Verification items for the finished model (mm, model axes). A direction names the side the tool comes from. Coordinates: 2 decimals unless noted, no trailing zeros. Write each loop counter-clockwise with the first axis right and the second up, starting at its lowest first coordinate (ties: lowest second). Pieces come first, ordered by that corner, then holes. Notation, with made-up numbers: M 29,-15.75 L 38,-15.75 A21 ccw 38,1.25 Z; hole C 70,29.5 d9. An arc over 180 degrees is marked long. Answer in a Markdown table with one row per item.
from build123d import *

# Parameters (mm, degrees)
SKETCH1_W           = 139.7
SKETCH1_H           = 12.7
BOSS_EXTRUDE1_DEPTH = 101.6
SKETCH2_W           = 12.7
SKETCH2_H           = 6.35
BOSS_EXTRUDE2_DEPTH = 19.05
CUT_EXTRUDE1_REACH  = 190.906
SKETCH3_R           = 5.207
SKETCH4_R           = 22.225
CUT_EXTRUDE2_DEPTH  = 11.43
CUT_EXTRUDE3_REACH  = 190.825
SKETCH5_R           = 1.7018
SKETCH5_R_2         = 2.2479
CUT_EXTRUDE4_REACH  = 187.568
SKETCH6_R           = 3.175
FILLET1_R           = 2.54


with BuildPart() as part:
    # Sketch1 → Boss-Extrude1 (new body)
    with BuildSketch(Plane(origin=(0, 0, 0), x_dir=(1, 0, 0), z_dir=(0, 1, 0))):
        with Locations((69.85, 6.35)):
            Rectangle(SKETCH1_W, SKETCH1_H)
    extrude(amount=BOSS_EXTRUDE1_DEPTH)

    # Sketch2 → Boss-Extrude2 (add)
    with BuildSketch(Plane.ZY):
        with Locations((-6.35, 3.175)):
            Rectangle(SKETCH2_W, SKETCH2_H)
    boss_extrude2 = extrude(amount=BOSS_EXTRUDE2_DEPTH)

    # Mirror1: Boss-Extrude2 across plane
    add(boss_extrude2.mirror(Plane.ZY.offset(-69.85)))

    # Sketch3 → Cut-Extrude1 (cut, up to next)
    with BuildSketch(Plane.XY, mode=Mode.PRIVATE) as cut_extrude1_sk1:
        with Locations((69.85, 76.2)):
            Circle(SKETCH3_R)
    cut_extrude1_tool1 = extrude(cut_extrude1_sk1.sketch, amount=-CUT_EXTRUDE1_REACH, mode=Mode.PRIVATE) & part.part
    add(cut_extrude1_tool1.solids().sort_by_distance((69.85, 76.2, 0))[0], mode=Mode.SUBTRACT)

    # Sketch4 → Cut-Extrude2 (cut)
    with BuildSketch(Plane.XY):
        with Locations((69.85, 76.2)):
            Circle(SKETCH4_R)
    extrude(amount=-CUT_EXTRUDE2_DEPTH, mode=Mode.SUBTRACT)

    # Sketch5 → Cut-Extrude3 (cut, up to next)
    with BuildSketch(Plane.XY.offset(-11.43), mode=Mode.PRIVATE) as cut_extrude3_sk1:
        with Locations((58.851477372, 82.55)):
            Circle(SKETCH5_R)
    cut_extrude3_tool1 = extrude(cut_extrude3_sk1.sketch, amount=-CUT_EXTRUDE3_REACH, mode=Mode.PRIVATE) & part.part
    # Sketch5 → Cut-Extrude3 (cut, up to next)
    with BuildSketch(Plane.XY.offset(-11.43), mode=Mode.PRIVATE) as cut_extrude3_sk2:
        with Locations((66.562998127, 88.467257994)):
            Circle(SKETCH5_R_2)
    cut_extrude3_tool2 = extrude(cut_extrude3_sk2.sketch, amount=-CUT_EXTRUDE3_REACH, mode=Mode.PRIVATE) & part.part
    # Sketch5 → Cut-Extrude3 (cut, up to next)
    with BuildSketch(Plane.XY.offset(-11.43), mode=Mode.PRIVATE) as cut_extrude3_sk3:
        with Locations((82.117257994, 79.487001873)):
            Circle(SKETCH5_R_2)
    cut_extrude3_tool3 = extrude(cut_extrude3_sk3.sketch, amount=-CUT_EXTRUDE3_REACH, mode=Mode.PRIVATE) & part.part
    # Sketch5 → Cut-Extrude3 (cut, up to next)
    with BuildSketch(Plane.XY.offset(-11.43), mode=Mode.PRIVATE) as cut_extrude3_sk4:
        with Locations((73.137001873, 63.932742006)):
            Circle(SKETCH5_R_2)
    cut_extrude3_tool4 = extrude(cut_extrude3_sk4.sketch, amount=-CUT_EXTRUDE3_REACH, mode=Mode.PRIVATE) & part.part
    # Sketch5 → Cut-Extrude3 (cut, up to next)
    with BuildSketch(Plane.XY.offset(-11.43), mode=Mode.PRIVATE) as cut_extrude3_sk5:
        with Locations((57.582742006, 72.912998127)):
            Circle(SKETCH5_R_2)
    cut_extrude3_tool5 = extrude(cut_extrude3_sk5.sketch, amount=-CUT_EXTRUDE3_REACH, mode=Mode.PRIVATE) & part.part
    # Sketch5 → Cut-Extrude3 (cut, up to next)
    with BuildSketch(Plane.XY.offset(-11.43), mode=Mode.PRIVATE) as cut_extrude3_sk6:
        with Locations((76.2, 87.198522628)):
            Circle(SKETCH5_R)
    cut_extrude3_tool6 = extrude(cut_extrude3_sk6.sketch, amount=-CUT_EXTRUDE3_REACH, mode=Mode.PRIVATE) & part.part
    # Sketch5 → Cut-Extrude3 (cut, up to next)
    with BuildSketch(Plane.XY.offset(-11.43), mode=Mode.PRIVATE) as cut_extrude3_sk7:
        with Locations((80.848522628, 69.85)):
            Circle(SKETCH5_R)
    cut_extrude3_tool7 = extrude(cut_extrude3_sk7.sketch, amount=-CUT_EXTRUDE3_REACH, mode=Mode.PRIVATE) & part.part
    # Sketch5 → Cut-Extrude3 (cut, up to next)
    with BuildSketch(Plane.XY.offset(-11.43), mode=Mode.PRIVATE) as cut_extrude3_sk8:
        with Locations((63.5, 65.201477372)):
            Circle(SKETCH5_R)
    cut_extrude3_tool8 = extrude(cut_extrude3_sk8.sketch, amount=-CUT_EXTRUDE3_REACH, mode=Mode.PRIVATE) & part.part
    add(cut_extrude3_tool1.solids().sort_by_distance((58.851477, 82.55, -11.43))[0], mode=Mode.SUBTRACT)
    add(cut_extrude3_tool2.solids().sort_by_distance((66.562998, 88.467258, -11.43))[0], mode=Mode.SUBTRACT)
    add(cut_extrude3_tool3.solids().sort_by_distance((82.117258, 79.487002, -11.43))[0], mode=Mode.SUBTRACT)
    add(cut_extrude3_tool4.solids().sort_by_distance((73.137002, 63.932742, -11.43))[0], mode=Mode.SUBTRACT)
    add(cut_extrude3_tool5.solids().sort_by_distance((57.582742, 72.912998, -11.43))[0], mode=Mode.SUBTRACT)
    add(cut_extrude3_tool6.solids().sort_by_distance((76.2, 87.198523, -11.43))[0], mode=Mode.SUBTRACT)
    add(cut_extrude3_tool7.solids().sort_by_distance((80.848523, 69.85, -11.43))[0], mode=Mode.SUBTRACT)
    add(cut_extrude3_tool8.solids().sort_by_distance((63.5, 65.201477, -11.43))[0], mode=Mode.SUBTRACT)

    # Sketch6 → Cut-Extrude4 (cut, up to next)
    with BuildSketch(Plane(origin=(0, 6.35, 0), x_dir=(1, 0, 0), z_dir=(0, 1, 0)), mode=Mode.PRIVATE) as cut_extrude4_sk1:
        with Locations(Location((-9.906, 6.35, 0), (0, 0, 270))):
            Circle(SKETCH6_R)
    cut_extrude4_tool1 = extrude(cut_extrude4_sk1.sketch, amount=-CUT_EXTRUDE4_REACH, mode=Mode.PRIVATE) & part.part
    cut_extrude4 = cut_extrude4_tool1.solids().sort_by_distance((-9.906, 6.35, -6.35))[0]
    add(cut_extrude4, mode=Mode.SUBTRACT)

    # Mirror2: Cut-Extrude4 across plane
    add(cut_extrude4.mirror(Plane.ZY.offset(-69.85)), mode=Mode.SUBTRACT)

    # Fillet1
    fillet1_edges = [part.edges().sort_by_distance(p)[0] for p in [
        (139.7, 101.6, -6.35),
        (-19.05, 6.35, -6.35),
        (158.75, 6.35, -6.35),
        (0, 101.6, -6.35),
    ]]
    fillet(fillet1_edges, radius=FILLET1_R)


solid = part.part
1) Tool access check on faces 1 (the face through (139.7, 52, -6)), 2 (the face through (74, 72, -11.43)), 3 (the face through (57.15, 82.62, -12.06)), 4 (the face through (0, 52, -6)). Record the directions out of +Z, -Z, +X, -X, +Y, -Y that give a thin tool (end or side, any length) a straight path to the whole face; none if there is none.
Response values:
| item | result |
|---|---|
| face 1 | +Z, -Z, +X, +Y |
| face 2 | +Z |
| face 3 | +Z, -Z |
| face 4 | +Z, -Z, -X, +Y |
2) Sectioned sample at B-B (y = 59). Record the cut outline in (x, z), then the cut area to 3 significant figures.
Response values:
| item | result |
|---|---|
| outline | M 0,-12.7 L 139.7,-12.7 L 139.7,0 L 83.93,0 L 83.93,-11.43 L 55.77,-11.43 L 55.77,0 L 0,0 Z |
| area | 1,450 mm² |
3) Sectioned sample at D-D (y = 19). Record the cut outline in (x, z).
Response values:
| item | result |
|---|---|
| outline | M 0,-12.7 L 139.7,-12.7 L 139.7,0 L 0,0 Z |
4) Thickness scan on L1, parallel to X at y = 69.85, z = -12; L2, parallel to X at y = 7.5, z = -9.25; L3, parallel to Y at x = -4, z = -7.75. Record the ranges inside material, lowest first. Write a range as [from, to].
Response values:
| item | result |
|---|---|
| L1 | x = [0, 79.15], [82.55, 139.7] |
| L2 | x = [0, 139.7] |
| L3 | y = [0, 6.35] |
5) Sectioned sample at C-C (x = 87.5). Record the cut outline in (y, z).
Response values:
| item | result |
|---|---|
| outline | M 0,-12.7 L 101.6,-12.7 L 101.6,0 L 89.71,0 L 89.71,-11.43 L 62.69,-11.43 L 62.69,0 L 0,0 Z |
6) Depth check by flat-ended pin: pin 1 (16.5 mm diameter, centred on x = 69.85, y = 76.2, fed in from +Z); pin 2 (2 mm diameter, centred on x = 76.2, y = 87.2, fed in from -Z); pin 3 (7.5 mm diameter, centred on x = 149.606, z = -6.35, fed in from +Y); pin 4 (1 mm diameter, centred on y = 13, z = -9, fed in from -X). Enter the tip coordinate at first touch or a pass-through.
Response values:
| item | result |
|---|---|
| pin 1 | stops at z = -11.43 |
| pin 2 | passes through |
| pin 3 | stops at y = 6.35 |
| pin 4 | stops at x = 0 |
7) Sectioned sample at A-A (z = -7.75). Record the cut outline in (x, y) (3 decimals).
Response values:
| item | result |
|---|---|
| outline | M -19.05,0 L -12.756,0 L -12.756,6.35 L -16.51,6.35 A2.54 ccw -19.05,3.81 Z; M -7.056,0 L 146.756,0 L 146.756,6.35 L 139.7,6.35 L 139.7,99.06 A2.54 ccw 137.16,101.6 L 2.54,101.6 A2.54 ccw 0,99.06 L 0,6.35 L -7.056,6.35 Z; M 152.456,0 L 158.75,0 L 158.75,3.81 A2.54 ccw 156.21,6.35 L 152.456,6.35 Z; hole C 69.85,76.2 d44.45 |
8) Release check for a two-part mould opening along Y. For faces 5 (the face through (-6, 6.35, -6)), 6 (the face through (158.75, 2, -6)), 7 (the face through (72.65, 61.74, -12.06)) record: +Y half, -Y half, draft (parallel to the pull), parting line (faces both ways), or undercut.
Response values:
| item | result |
|---|---|
| face 5 | +Y half |
| face 6 | draft |
| face 7 | undercut |
